from build123d import *

# Parameters (mm, degrees)
EXTRUSION1_DEPTH             = 200
ENL_V_MAT_EXTRU_1_DEPTH      = 319.955094772
ENL_V_MAT_EXTRU_1_DEPTH_BACK = 319.955094772
ESQUISSE4_OUTSIDE_W          = 486.616
ESQUISSE4_OUTSIDE_H          = 292.116
COQUE5_T                     = 6
ENL_V_MAT_EXTRU_2_DEPTH      = 292.26680635
ENL_V_MAT_EXTRU_2_DEPTH_BACK = 292.26680635
ESQUISSE5_W                  = 100
ESQUISSE5_H                  = 45
ESQUISSE6_R                  = 10
ENL_V_MAT_EXTRU_3_DEPTH      = 270.348013695
ESQUISSE7_R                  = 10
ENL_V_MAT_EXTRU_4_DEPTH      = 270.348013695


with BuildPart() as part:
    # Esquisse2 → Extrusion1 (new body)
    with BuildSketch(Plane.XY):
        with BuildLine():
            Line((-105.570349674, 42.982720814), (211.674532216, 33.986337388))
            ThreePointArc((211.674532216, 33.986337388), (244.710752688, 0), (211.674532216, -33.986337388))
            Line((211.674532216, -33.986337388), (-105.570349674, -42.982720814))
            ThreePointArc((-105.570349674, -42.982720814), (-149.789247312, 0), (-105.570349674, 42.982720814))
        make_face()
    extrude(amount=EXTRUSION1_DEPTH)

    # Esquisse4 outside → Enlèv. mat.-Extru.1 (cut, two sides: drawn at the far end of the back side and taken through both)
    with BuildSketch(Plane(origin=(0, 0, 0), x_dir=(1, 0, 0), z_dir=(0, 1, 0)).offset(-ENL_V_MAT_EXTRU_1_DEPTH_BACK)):
        with Locations((47.461, -100)):
            Rectangle(ESQUISSE4_OUTSIDE_W, ESQUISSE4_OUTSIDE_H)
        Polygon((-158.789247312, -152), (-158.789247312, -48), (-91.789247312, -48), (311.210752688, -72), (311.210752688, -128), (-91.789247312, -152), align=None, mode=Mode.SUBTRACT)
    extrude(amount=ENL_V_MAT_EXTRU_1_DEPTH + ENL_V_MAT_EXTRU_1_DEPTH_BACK, mode=Mode.SUBTRACT)

    # Coque5 (no face opened: a closed hollow body)
    add(offset(amount=-COQUE5_T, mode=Mode.PRIVATE), mode=Mode.SUBTRACT)

    # Esquisse5 → Enlèv. mat.-Extru.2 (cut, two sides: drawn at the far end of the back side and taken through both)
    with BuildSketch(Plane(origin=(0, 0, 0), x_dir=(1, 0, 0), z_dir=(0, 1, 0)).offset(-ENL_V_MAT_EXTRU_2_DEPTH_BACK)):
        with Locations((223.210752688, -102.5)):
            Rectangle(ESQUISSE5_W, ESQUISSE5_H)
    extrude(amount=ENL_V_MAT_EXTRU_2_DEPTH + ENL_V_MAT_EXTRU_2_DEPTH_BACK, mode=Mode.SUBTRACT)

    # Esquisse6 → Enlèv. mat.-Extru.3 (cut, through all)
    with BuildSketch(Plane.XY.offset(152)):
        with Locations((210.710752688, 0)):
            Circle(ESQUISSE6_R)
    extrude(amount=-ENL_V_MAT_EXTRU_3_DEPTH, mode=Mode.SUBTRACT)

    # Esquisse7 → Enlèv. mat.-Extru.4 (cut, through all)
    with BuildSketch(Plane.XY.offset(152)):
        with Locations((-106.789247312, 0)):
            Circle(ESQUISSE7_R)
    extrude(amount=-ENL_V_MAT_EXTRU_4_DEPTH, mode=Mode.SUBTRACT)


solid = part.part
Geometry: final body of the model. Coordinates: model frame, mm. A direction names the side the tool comes from. Give positions to 0.01 mm unless a question says otherwise; leave off trailing zeros. Write each loop counter-clockwise with the first axis right and the second up, starting at its lowest first coordinate (ties: lowest second). Pieces come first, ordered by that corner, then holes. Notation, with made-up numbers: M -1.5,35 L 7.5,35 A32 cw 7.5,71 Z; hole C 64,11.25 d10. An arc over 180 degrees is marked long. Answer in a Markdown table with one row per item. Add a question column.
(1) Section B-B on z = 117.5. Return loops of the section in (x, y).
(2) Section D-D on y = 16. Return loops of the section in (x, z).
(3) Section A-A on y = 0. State how many separate pieces and enclosed holes the cut face has, and give its area (3 significant figures).
(4) Section C-C on x = -31. Return loops of the section in (y, z), and give its area (3 significant figures).
(5) Mould query, pull axis Y, two halves, no side actions, for faces 1 (the cylindrical face through (200.72, 0.44, 131.06)), 2 (the cylindrical face through (-149.78, -0.96, 99.27)), 3 (the flat face through (238, 8, 80)), 4 (the cylindrical face through (238.704, 0.605, 76.862)). Classes: +Y half, -Y half, draft (parallel to the pull), parting line (faces both ways), or undercut.
(6) First-contact query: pin 1 (1.5 mm diameter, centred on x = 96, y = -15, fed in from -Z); pin 2 (6 mm diameter, centred on y = -6, z = 121.5, fed in from -X); pin 3 (6 mm diameter, centred on x = 132, y = -12.5, fed in from -Z). Flat tips, straight axial feed; report the tip coordinate or a pass-through.
(7) Ray query, line 1 (Y direction, x = -72, z = 121.5); line 2 (Z direction, x = -47, y = 27); line 3 (Y direction, x = 117.5, z = 126). Return the intervals inside material, ascending.
(8) Reachability of faces 5 (the flat face through (-118, -1, 146)), 6 (the flat face through (238, 8, 125)), 7 (the cylindrical face through (244.703, 0.734, 72.939)) from +Z, -Z, +X, -X, +Y, -Y: full face, straight path, thin tool, end or side. Return the list, or none.
Result set:
| question | item | result |
|---|---|---|
| 1 | outline | M -105.74,-36.99 A37 cw long -105.74,36.99 L 173.21,29.07 L 173.21,35.08 L -105.57,42.98 A43 ccw long -105.57,-42.98 L 173.21,-35.08 L 173.21,-29.07 Z |
| 2 | outline | M -146.7,48 L -91.79,48 L 240.71,67.8 L 240.71,80 L 233.69,80 L 233.69,73.39 L -91.97,54 L -140.15,54 L -140.15,146 L -91.97,146 L 233.69,126.61 L 233.69,125 L 240.71,125 L 240.71,132.2 L -91.79,152 L -146.7,152 Z |
| 3 | separate pieces | 5 |
| 3 | enclosed holes | 0 |
| 3 | area | 4,860 mm^2 |
| 4 | outline | M -40.87,51.62 L 40.87,51.62 L 40.87,148.38 L -40.87,148.38 Z; hole M -34.87,57.63 L 34.87,57.63 L 34.87,142.37 L -34.87,142.37 Z |
| 4 | area | 2,000 mm^2 |
| 5 | face 1 | undercut |
| 5 | face 2 | parting line |
| 5 | face 3 | draft |
| 5 | face 4 | undercut |
| 6 | pin 1 | stops at z = 59.14 |
| 6 | pin 2 | stops at x = -149.68 |
| 6 | pin 3 | stops at z = 61.15 |
| 7 | line 1 | y = -42.03 to -36.03, 36.03 to 42.03 |
| 7 | line 2 | z = 50.67 to 56.68, 143.32 to 149.33 |
| 7 | line 3 | y = -36.66 to -30.65, 30.65 to 36.66 |
| 8 | face 5 | none |
| 8 | face 6 | +X, +Y, -Y |
| 8 | face 7 | +Z, -Z, +X |
